```python
from build123d import *

# Parameters (mm, degrees)
F1_DEPTH = 20
F3_T     = 2
F4_R     = 1.99999


# Not quite as in the source:
# - a fillet or chamfer is up to 0.001 mm smaller than in the source, because OpenCascade refuses the exact size
# - a feature of the source that left no trace in its solid (it failed there, or was rolled back) is left out
# - a shell that OpenCascade refuses in one call is made with other operations: the cavity is built on its own and cut out


with BuildPart() as f1:
    # F0 (on Top) → F1 (new body)
    with BuildSketch(Plane.XY):
        with BuildLine():
            Line((-8, -10), (8, -10))
            ThreePointArc((8, -10), (9.4142135624, -9.4142135624), (10, -8))
            Line((10, -8), (10, 8))
            ThreePointArc((10, 8), (9.4142135624, 9.4142135624), (8, 10))
            Line((8, 10), (-8, 10))
            ThreePointArc((-8, 10), (-9.4142135624, 9.4142135624), (-10, 8))
            Line((-10, 8), (-10, -8))
            ThreePointArc((-10, -8), (-9.4142135624, -9.4142135624), (-8, -10))
        make_face()
    extrude(amount=F1_DEPTH)

    # F3: shell of thickness 2, made by hand


with BuildPart() as f3_core1:
    # F3_t2: copy of F1
    add(f1.part)

    # the walls: a layer under each face that stays
    f3_faces = [f3_core1.faces().sort_by_distance(p)[0] for p in [
        (0, -10, 10),
        (10, 0, 10),
        (0, 10, 10),
        (-10, 0, 10),
        (0, 0, 0),
    ]]
    thicken(f3_faces, amount=-F3_T, mode=Mode.SUBTRACT)


with BuildPart() as f1_1:
    add(f1.part)

    # what is left inside the walls is the cavity
    f3_cavity = [f3_core1.part.solids().sort_by_distance(p)[0] for p in [
        (0, -7.98, 14),
    ]]
    add(f3_cavity, mode=Mode.SUBTRACT)

    # F4 (radius 2 in the source; OpenCascade refuses exactly that, so slightly less here)
    f4_edges = [f1_1.edges().sort_by_distance(p)[0] for p in [
        (0, -10, 0),
        (0, -10, 20),
        (-9.414214, -9.414214, 0),
        (-9.414214, -9.414214, 20),
        (9.414214, -9.414214, 0),
        (9.414214, -9.414214, 20),
        (10, 0, 0),
        (9.414214, 9.414214, 0),
        (0, 10, 0),
        (-9.414214, 9.414214, 0),
        (-10, 0, 0),
        (-10, 0, 20),
        (10, 0, 20),
        (-9.414214, 9.414214, 20),
        (9.414214, 9.414214, 20),
        (0, 10, 20),
        (0, -8, 2),
        (8, 0, 2),
        (0, 8, 2),
        (-8, 0, 2),
    ]]
    fillet(f4_edges, radius=F4_R)


solid = f1_1.part
```
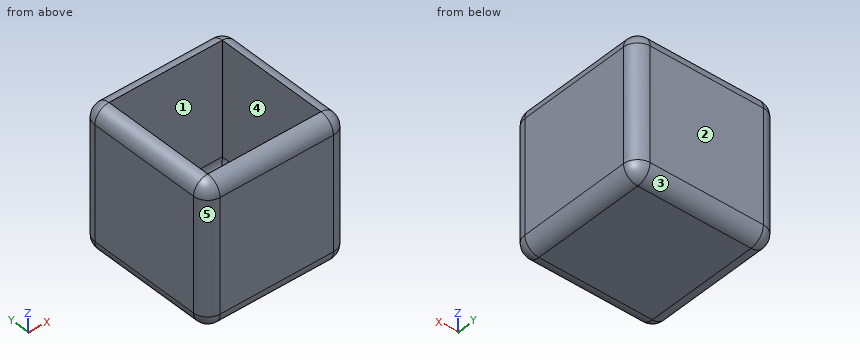
Source: CAD feature listing. Evaluate the final solid. Frame: model axes, mm. Face numbers are marked on the shaded views. A direction names the side the tool comes from. Give positions to 0.01 mm unless a question says otherwise; leave off trailing zeros. Loops run counter-clockwise (first coordinate to the right, second up) from the corner with the lowest first, then second, coordinate; pieces in that order, holes last. Notation, with made-up numbers: (14, 32.25) -> (33, 32.25) arc R13 cw to (33, 40.25) -> close; hole circle Ø8 at (-10, 15.5). An arc over 180 degrees is marked (long way). Put each result on its own line as item: value. Start each with the question number.
1) Cut plane D-D (z = 2.75). Return loops of the section in (x, y), then the cut area to 3 significant figures.
2) Reachability of the marked faces 1 and 2 from +Z, -Z, +X, -X, +Y, -Y: full face, straight path, thin tool, end or side. Return the list, or none.
3) Material intervals for probe 1 along X at (y, z) = (-6.25, 16.5); probe 2 along Z at (x, y) = (1.25, 5.25), sorted ascending.
4) Contact query for flat-ended pins moving along their axis: P1, Ø3, axis at x = 0.5, y = 1.5, coming from the +Z side; P2, Ø9.5, axis at x = -0.5, y = 2.5, coming from the +Z side. Output: stop coordinate, or through.
5) Cut plane A-A (z = 16). Return loops of the section in (x, y).
6) Draft query along X for the marked faces 3, 4 and 5. Return one class per face: released by +X, released by -X, zero draft, split by the parting line, or undercut.
Results are:
1. outline: (-10, -8) arc R2 ccw to (-8, -10) -> (8, -10) arc R2 ccw to (10, -8) -> (10, 8) arc R2 ccw to (8, 10) -> (-8, 10) arc R2 ccw to (-10, 8) -> close; hole (-7.56, -7.56) -> (7.56, -7.56) -> (7.56, 7.56) -> (-7.56, 7.56) -> close
1. area: 168 mm2
2. face 1: +Z
2. face 2: +Z, -Z, +X, -X, +Y
3. probe 1: x = -10 to -8, 8 to 10
3. probe 2: z = 0 to 2
4. P1: stops at z = 2
4. P2: stops at z = 2.44
5. outline: (-10, -8) arc R2 ccw to (-8, -10) -> (8, -10) arc R2 ccw to (10, -8) -> (10, 8) arc R2 ccw to (8, 10) -> (-8, 10) arc R2 ccw to (-10, 8) -> close; hole (-8, -8) -> (8, -8) -> (8, 8) -> (-8, 8) -> close
6. face 3: zero draft
6. face 4: undercut
6. face 5: released by -X
